Could you check a few things on this model? Use its own coordinates, in mm. Face numbers are marked on the shaded views. Coordinates: 2 decimals unless noted, no trailing zeros.
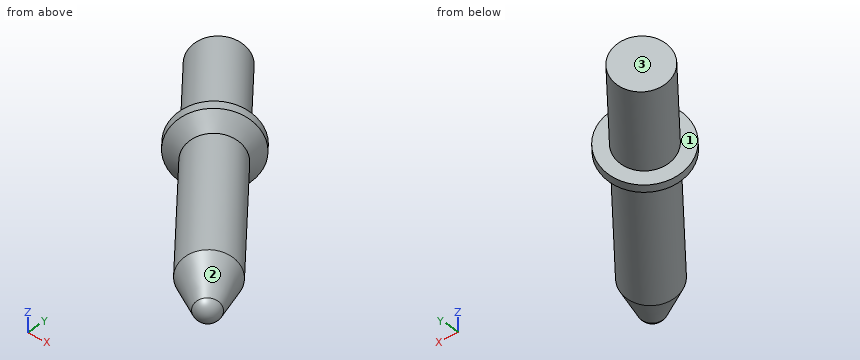
```python
from build123d import *


with BuildPart() as part:
    # Sketch2 → Revolve1 (revolve)
    with BuildSketch(Plane.XY):
        with BuildLine():
            Line((25.047699583, 26.952680264), (36.149927178, 13.721560642))
            Line((36.149927178, 13.721560642), (37.97893489, 15.256280339))
            Line((37.97893489, 15.256280339), (39.007523623, 14.030456021))
            Line((39.007523623, 14.030456021), (38.713235608, 10.666728612))
            Line((38.713235608, 10.666728612), (55.059298025, -8.813749999))
            Line((55.059298025, -8.813749999), (57.671314579, -15.990206501))
            ThreePointArc((57.671314579, -15.990206501), (57.731349183, -17.365224991), (56.991848446, -18.526008632))
            Line((56.991848446, -18.526008632), (21.399412923, 23.891404273))
            Line((21.399412923, 23.891404273), (25.047699583, 26.952680264))
        make_face()
    revolve(axis=Axis((56.991848446, -18.526008632, 0), (-0.6427876096865393, 0.7660444431189782, 0)))


solid = part.part
```
1. If we mould it in two halves opening along X, with no side actions, what happens to the marked faces 1, 2 and 3? For each: pulls with the +X half, pulls with the -X half, needs draft (parallel to the pull), parting line crosses it, or undercut.
Verdict:
face 1: undercut
face 2: parting line crosses it
face 3: pulls with the -X half
2. For pin 1 (4 mm diameter, centred on x = 48, z = -0.5, fed in from +Y); pin 2 (4 mm diameter, centred on x = 28.5, z = -4, fed in from -Y); pin 3 (5 mm diameter, centred on x = 42.5, z = -3.5, fed in from -Y), each with a flat end and sliding along its axis, tell me the tip position at first contact or that it passes through.
Verdict:
pin 1: stops at y = 1.96
pin 2: stops at y = 4.99
pin 3: stops at y = -10.37
3. Please list where these lines run through material, in increasing order: line 1 along X through (y, z) = (14.5, -1.75); line 2 along Y through (x, z) = (27.5, 2); line 3 along Z through (x, y) = (30.5, 19).
Verdict:
line 1: x = 23.5 to 35.06, 37.08 to 38.33
line 2: y = 5.94 to 6.46, 9.9 to 23.35
line 3: z = -2.83 to 2.83
